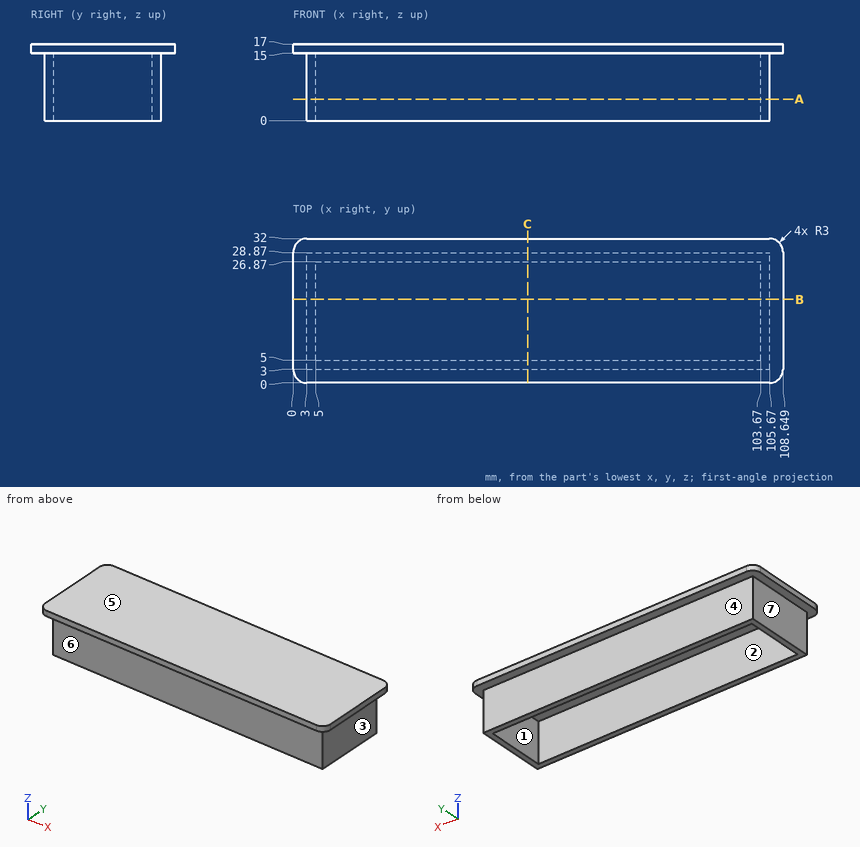
Verification items for this drawing (mm, ordinates from the low corner). A direction names the side the tool comes from. Give positions to 0.01 mm unless a question says otherwise; leave off trailing zeros. Loops run counter-clockwise (first coordinate to the right, second up) from the corner with the lowest first, then second, coordinate; pieces in that order, holes last.
(1) Set-up check for the marked faces 5, 6 and 7: record each of +Z, -Z, +X, -X, +Y, -Y from which the full face is reachable in a straight line by a thin tool's end or side.
From the geometry:
face 5: +Z, +X, -X, +Y, -Y
face 6: -Z, +X, -X, -Y
face 7: -Z, -X, +Y, -Y
(2) Section check C-C on x = 52. Record the cut outline in (y, z).
From the geometry:
outline: (0, 15) - (3, 15) - (3, 0) - (5, 0) - (5, 15) - (26.87, 15) - (26.87, 0) - (28.87, 0) - (28.87, 15) - (32, 15) - (32, 17) - (0, 17) - close
(3) Release check for a two-part mould opening along X. For the marked faces 1, 2, 3 and 4 record: released by +X, released by -X, zero draft, split by the parting line, or undercut.
From the geometry:
face 1: undercut
face 2: undercut
face 3: released by +X
face 4: zero draft
(4) Section check B-B on y = 18.5. Record the cut outline in (x, z), then the cut area to 3 significant figures.
From the geometry:
outline: (0, 15) - (3, 15) - (3, 0) - (5, 0) - (5, 15) - (103.67, 15) - (103.67, 0) - (105.67, 0) - (105.67, 15) - (108.65, 15) - (108.65, 17) - (0, 17) - close
area: 277 mm2
(5) Depth check by flat-ended pin: pin 1 Ø2 at (x, z) = (74.5, 9) entering from -Y; pin 2 Ø8 at (x, y) = (37, 21.5) entering from -Z; pin 3 Ø1.5 at (y, z) = (13.5, 2.5) entering from +X. Enter the tip coordinate at first touch or a pass-through.
From the geometry:
pin 1: stops at y = 3
pin 2: stops at z = 15
pin 3: stops at x = 105.67
(6) Section check A-A on z = 4.75. Record the cut outline in (x, y), then the cut area to 3 significant figures.
From the geometry:
outline: (3, 3) - (105.67, 3) - (105.67, 28.87) - (3, 28.87) - close; hole (5, 5) - (103.67, 5) - (103.67, 26.87) - (5, 26.87) - close
area: 498 mm2
(7) Thickness scan on L1, parallel to X at y = 25.5, z = 13.25; L2, parallel to Y at x = 102, z = 9.25; L3, parallel to Z at x = 25.5, y = 24. Record the ranges inside material, lowest first.
From the geometry:
L1: x = 3 to 5, 103.67 to 105.67
L2: y = 3 to 5, 26.87 to 28.87
L3: z = 15 to 17
